Source: CAD feature listing. Evaluate the final solid. Frame: model axes, mm. Face numbers are marked on the shaded views. A direction names the side the tool comes from. Round coordinates to 2 decimals unless told otherwise and drop trailing zeros. Order: outer loops, then holes, each group sorted by start corner. A loop starts at its lowest first (then second) coordinate and runs counter-clockwise, first axis right, second up. Notation, with made-up numbers: (-17, 10) -> (4, 10) arc R25 cw to (4, 28) -> close; hole circle Ø5 at (-29.5, 39). An arc over 180 degrees is marked (long way). Answer as CSV lines item,"result".
from build123d import *

# Parameters (mm, degrees)
SKETCH1_W           = 132
SKETCH1_H           = 72
BOSS_EXTRUDE1_DEPTH = 47.625
CUT_EXTRUDE1_START  = -95.25
CUT_EXTRUDE1_DEPTH  = 95.25
SKETCH3_W           = 96
SKETCH3_H           = 38.1
CUT_EXTRUDE2_DEPTH  = 109.665268715
SKETCH4_R           = 15
CUT_EXTRUDE3_DEPTH  = 145.656822687
BOSS_EXTRUDE2_START = 16
SKETCH5_R           = 36
SKETCH5_R_2         = 15
BOSS_EXTRUDE2_DEPTH = 16
SKETCH6_R           = 12
CUT_EXTRUDE4_DEPTH  = 131.738527221


# Read off the part's stored shape, not the designer's step: Cut-Extrude1
with BuildPart() as part:
    # Sketch1 → Boss-Extrude1 (new, symmetric)
    with BuildSketch(Plane.XY):
        Rectangle(SKETCH1_W, SKETCH1_H)
    extrude(amount=BOSS_EXTRUDE1_DEPTH, both=True)

    # Cut-Extrude1 outline → Cut-Extrude1 (cut)
    with BuildSketch(Plane.XY.offset(47.625).offset(CUT_EXTRUDE1_START)):
        with BuildLine():
            Line((-66, -36), (-29.762876885, -36))
            ThreePointArc((-29.762876885, -36), (-65.762876885, 0), (-29.762876885, 36))
            Line((-29.762876885, 36), (-66, 36))
            Line((-66, 36), (-66, -36))
        make_face()
    extrude(amount=CUT_EXTRUDE1_DEPTH, mode=Mode.SUBTRACT)

    # Sketch3 → Cut-Extrude2 (cut, through all)
    with BuildSketch(Plane.XZ.offset(36)):
        with Locations((-17.762876885, -0.395)):
            Rectangle(SKETCH3_W, SKETCH3_H)
    extrude(amount=-CUT_EXTRUDE2_DEPTH, mode=Mode.SUBTRACT)

    # Sketch4 → Cut-Extrude3 (cut, through all)
    with BuildSketch(Plane(origin=(66, 0, 0), x_dir=(0, 0, -1), z_dir=(1, 0, 0))):
        with Locations(Location((0, 0, 0), (0, 0, 90))):
            Circle(SKETCH4_R)
    extrude(amount=-CUT_EXTRUDE3_DEPTH, mode=Mode.SUBTRACT)

    # Sketch5 → Boss-Extrude2 (add)
    with BuildSketch(Plane(origin=(66, 0, 0), x_dir=(0, 0, -1), z_dir=(1, 0, 0)).offset(BOSS_EXTRUDE2_START)):
        with Locations(Location((0, 0, 0), (0, 0, 90))):
            Circle(SKETCH5_R)
        with Locations(Location((0, 0, 0), (0, 0, 90))):
            Circle(SKETCH5_R_2, mode=Mode.SUBTRACT)
    extrude(amount=-BOSS_EXTRUDE2_DEPTH)

    # Sketch6 → Cut-Extrude4 (cut, through all)
    with BuildSketch(Plane(origin=(0, 0, -47.625), x_dir=(-1, 0, 0), z_dir=(0, 0, -1))):
        with Locations((31.598726765, 0)):
            Circle(SKETCH6_R)
    extrude(amount=-CUT_EXTRUDE4_DEPTH, mode=Mode.SUBTRACT)


solid = part.part
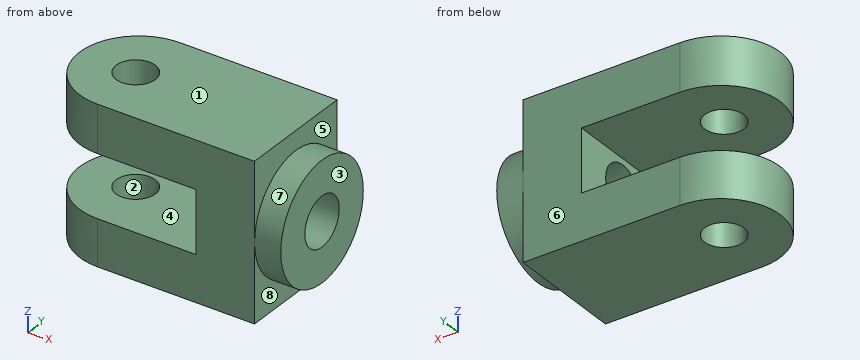
1. Pin query (flat end, axial travel): pin 1 (18 mm diameter, centred on y = 0, z = 0, fed in from -X); pin 2 (1 mm diameter, centred on x = -36.5, z = -27, fed in from +Y); pin 3 (4 mm diameter, centred on y = 25.5, z = -26, fed in from -X). Return the tip coordinate at first contact, or that it passes through.
Results below:
pin 1,"through"
pin 2,"y = 35.46"
pin 3,"x = -57.03"
2. Mould query, pull axis X, two halves, no side actions, for the marked faces 1, 2 and 3. Classes: released by +X, released by -X, zero draft, split by the parting line, or undercut.
Results below:
face 1,"zero draft"
face 2,"undercut"
face 3,"released by +X"
3. Section query D-D on z = 11.5. Return loops of the section in (x, y), and give its area (3 significant figures).
Results below:
outline,"(30.24, -36) -> (66, -36) -> (66, -34.11) -> (82, -34.11) -> (82, -9.63) -> (30.24, -9.63) -> close; (30.24, 9.63) -> (82, 9.63) -> (82, 34.11) -> (66, 34.11) -> (66, 36) -> (30.24, 36) -> close"
area,"2,670 mm2"
4. Section query B-B on x = 64. Return loops of the section in (y, z) (3 decimals).
Results below:
outline,"(-36, -47.625) -> (36, -47.625) -> (36, 47.625) -> (-36, 47.625) -> close; hole circle Ø30 at (0, 0)"
5. Section query C-C on z = -30. Return loops of the section in (x, y), and give its area (3 significant figures).
Results below:
outline,"(-29.76, -36) -> (66, -36) -> (66, -19.9) -> (82, -19.9) -> (82, 19.9) -> (66, 19.9) -> (66, 36) -> (-29.76, 36) arc R36 ccw to start; hole circle Ø24 at (-31.6, 0)"
area,"9,120 mm2"
6. Reachability of the marked faces 4, 5, 6, 7 and 8 from +Z, -Z, +X, -X, +Y, -Y: full face, straight path, thin tool, end or side. Return the list, or none.
Results below:
face 4,"-X, +Y, -Y"
face 5,"+Z, +X"
face 6,"+Z, -Z, +X, -X, +Y"
face 7,"+X"
face 8,"-Z, +X"
7. Line query: L1, parallel to Z at x = 28, y = 9 (3 decimals); L2, parallel to Z at x = 57, y = 0 (3 decimals); L3, parallel to X at y = -4.5, z = 18.5. Output: solid intervals per line, ascending. Write a range as [from, to].
Results below:
L1,"[-47.625, -19.445], [18.655, 47.625]"
L2,"[-47.625, -15], [15, 47.625]"
L3,"[30.24, 82]"
8. Section query A-A on y = 0. Return loops of the section in (x, z) (3 decimals), and give its area (3 significant figures).
Results below:
outline,"(-65.763, -47.625) -> (-43.599, -47.625) -> (-43.599, -19.445) -> (-65.763, -19.445) -> close; (-65.763, 18.655) -> (-43.599, 18.655) -> (-43.599, 47.625) -> (-65.763, 47.625) -> close; (-19.599, -47.625) -> (66, -47.625) -> (66, -36) -> (82, -36) -> (82, -15) -> (30.237, -15) -> (30.237, -19.445) -> (-19.599, -19.445) -> close; (-19.599, 18.655) -> (30.237, 18.655) -> (30.237, 15) -> (82, 15) -> (82, 36) -> (66, 36) -> (66, 47.625) -> (-19.599, 47.625) -> close"
area,"7,120 mm2"
